from build123d import *

# Parameters (mm, degrees)
BOSS_EXTRUDE1_START  = 46
SKETCH1_W            = 40
SKETCH1_H            = 10
BOSS_EXTRUDE1_DEPTH  = 28
BOSS_EXTRUDE2_START  = 48.4
SKETCH2_W            = 35.2
SKETCH2_H            = 12
BOSS_EXTRUDE2_DEPTH  = 23.2
BOSS_EXTRUDE3_START  = 50
SKETCH3_R            = 3
BOSS_EXTRUDE3_DEPTH  = 10
BOSS_EXTRUDE4_START  = 50
SKETCH4_R            = 3
BOSS_EXTRUDE4_DEPTH  = 10
BOSS_EXTRUDE5_START  = 50
SKETCH5_R            = 3
BOSS_EXTRUDE5_DEPTH  = 10
BOSS_EXTRUDE6_START  = 50
SKETCH6_R            = 3
BOSS_EXTRUDE6_DEPTH  = 10
BOSS_EXTRUDE7_START  = 50
SKETCH7_R            = 3
BOSS_EXTRUDE7_DEPTH  = 10
BOSS_EXTRUDE8_START  = 50
SKETCH8_R            = 3
BOSS_EXTRUDE8_DEPTH  = 10
BOSS_EXTRUDE9_START  = 50
SKETCH9_R            = 3
BOSS_EXTRUDE9_DEPTH  = 10
BOSS_EXTRUDE10_START = 50
SKETCH10_R           = 3
BOSS_EXTRUDE10_DEPTH = 10
BOSS_EXTRUDE11_START = 49
SKETCH11_R           = 1
BOSS_EXTRUDE11_DEPTH = 9.5
BOSS_EXTRUDE12_START = 49
SKETCH12_R           = 1
BOSS_EXTRUDE12_DEPTH = 9.5
BOSS_EXTRUDE13_START = 49
SKETCH13_R           = 1
BOSS_EXTRUDE13_DEPTH = 9.5
BOSS_EXTRUDE14_START = 49
SKETCH14_R           = 1
BOSS_EXTRUDE14_DEPTH = 9.5
BOSS_EXTRUDE15_START = 51.5
SKETCH15_R           = 1
BOSS_EXTRUDE15_DEPTH = 9.5
BOSS_EXTRUDE16_START = 51.5
SKETCH16_R           = 1
BOSS_EXTRUDE16_DEPTH = 9.5
BOSS_EXTRUDE17_START = 51.5
SKETCH17_R           = 1
BOSS_EXTRUDE17_DEPTH = 9.5
BOSS_EXTRUDE18_START = 51.5
SKETCH18_R           = 1
BOSS_EXTRUDE18_DEPTH = 9.5


with BuildPart() as part:
    # Sketch1 → Boss-Extrude1 (new body)
    with BuildSketch(Plane.XY.offset(BOSS_EXTRUDE1_START)):
        with Locations((0, 55)):
            Rectangle(SKETCH1_W, SKETCH1_H)
    extrude(amount=BOSS_EXTRUDE1_DEPTH)


with BuildPart() as body_2:
    # Sketch2 → Boss-Extrude2 (new body)
    with BuildSketch(Plane.XY.offset(BOSS_EXTRUDE2_START)):
        with Locations((0, 55)):
            Rectangle(SKETCH2_W, SKETCH2_H)
    extrude(amount=BOSS_EXTRUDE2_DEPTH)


with BuildPart() as part_1:
    add(part.part)

    # Combine1: cut body 2
    add(body_2.part, mode=Mode.SUBTRACT)

    # Sketch3 → Boss-Extrude3 (add)
    with BuildSketch(Plane(origin=(0, 0, 0), x_dir=(1, 0, 0), z_dir=(0, 1, 0)).offset(BOSS_EXTRUDE3_START)):
        with Locations((-15, -50.5)):
            Circle(SKETCH3_R)
    extrude(amount=BOSS_EXTRUDE3_DEPTH)

    # Sketch4 → Boss-Extrude4 (add)
    with BuildSketch(Plane(origin=(0, 0, 0), x_dir=(1, 0, 0), z_dir=(0, 1, 0)).offset(BOSS_EXTRUDE4_START)):
        with Locations((-15, -69.5)):
            Circle(SKETCH4_R)
    extrude(amount=BOSS_EXTRUDE4_DEPTH)

    # Sketch5 → Boss-Extrude5 (add)
    with BuildSketch(Plane(origin=(0, 0, 0), x_dir=(1, 0, 0), z_dir=(0, 1, 0)).offset(BOSS_EXTRUDE5_START)):
        with Locations((15, -50.5)):
            Circle(SKETCH5_R)
    extrude(amount=BOSS_EXTRUDE5_DEPTH)

    # Sketch6 → Boss-Extrude6 (add)
    with BuildSketch(Plane(origin=(0, 0, 0), x_dir=(1, 0, 0), z_dir=(0, 1, 0)).offset(BOSS_EXTRUDE6_START)):
        with Locations((15, -69.5)):
            Circle(SKETCH6_R)
    extrude(amount=BOSS_EXTRUDE6_DEPTH)

    # Sketch7 → Boss-Extrude7 (add)
    with BuildSketch(Plane(origin=(0, 0, 0), x_dir=(1, 0, 0), z_dir=(0, 1, 0)).offset(BOSS_EXTRUDE7_START)):
        with Locations((-6, -50)):
            Circle(SKETCH7_R)
    extrude(amount=BOSS_EXTRUDE7_DEPTH)

    # Sketch8 → Boss-Extrude8 (add)
    with BuildSketch(Plane(origin=(0, 0, 0), x_dir=(1, 0, 0), z_dir=(0, 1, 0)).offset(BOSS_EXTRUDE8_START)):
        with Locations((-6, -70)):
            Circle(SKETCH8_R)
    extrude(amount=BOSS_EXTRUDE8_DEPTH)

    # Sketch9 → Boss-Extrude9 (add)
    with BuildSketch(Plane(origin=(0, 0, 0), x_dir=(1, 0, 0), z_dir=(0, 1, 0)).offset(BOSS_EXTRUDE9_START)):
        with Locations((6, -50)):
            Circle(SKETCH9_R)
    extrude(amount=BOSS_EXTRUDE9_DEPTH)

    # Sketch10 → Boss-Extrude10 (add)
    with BuildSketch(Plane(origin=(0, 0, 0), x_dir=(1, 0, 0), z_dir=(0, 1, 0)).offset(BOSS_EXTRUDE10_START)):
        with Locations((6, -70)):
            Circle(SKETCH10_R)
    extrude(amount=BOSS_EXTRUDE10_DEPTH)


with BuildPart() as body_2_2:
    # Sketch11 → Boss-Extrude11 (new body)
    with BuildSketch(Plane(origin=(0, 0, 0), x_dir=(1, 0, 0), z_dir=(0, 1, 0)).offset(BOSS_EXTRUDE11_START)):
        with Locations(Location((-15, -50.5, 0), (0, 0, 270))):
            Circle(SKETCH11_R)
    extrude(amount=BOSS_EXTRUDE11_DEPTH)


with BuildPart() as part_2:
    add(part_1.part)

    # Combine2: cut body 2 2
    add(body_2_2.part, mode=Mode.SUBTRACT)


with BuildPart() as body_2_3:
    # Sketch12 → Boss-Extrude12 (new body)
    with BuildSketch(Plane(origin=(0, 0, 0), x_dir=(1, 0, 0), z_dir=(0, 1, 0)).offset(BOSS_EXTRUDE12_START)):
        with Locations(Location((-15, -69.5, 0), (0, 0, 270))):
            Circle(SKETCH12_R)
    extrude(amount=BOSS_EXTRUDE12_DEPTH)


with BuildPart() as part_3:
    add(part_2.part)

    # Combine3: cut body 2 3
    add(body_2_3.part, mode=Mode.SUBTRACT)


with BuildPart() as body_2_4:
    # Sketch13 → Boss-Extrude13 (new body)
    with BuildSketch(Plane(origin=(0, 0, 0), x_dir=(1, 0, 0), z_dir=(0, 1, 0)).offset(BOSS_EXTRUDE13_START)):
        with Locations(Location((15, -50.5, 0), (0, 0, 270))):
            Circle(SKETCH13_R)
    extrude(amount=BOSS_EXTRUDE13_DEPTH)


with BuildPart() as part_4:
    add(part_3.part)

    # Combine4: cut body 2 4
    add(body_2_4.part, mode=Mode.SUBTRACT)


with BuildPart() as body_2_5:
    # Sketch14 → Boss-Extrude14 (new body)
    with BuildSketch(Plane(origin=(0, 0, 0), x_dir=(1, 0, 0), z_dir=(0, 1, 0)).offset(BOSS_EXTRUDE14_START)):
        with Locations(Location((15, -69.5, 0), (0, 0, 270))):
            Circle(SKETCH14_R)
    extrude(amount=BOSS_EXTRUDE14_DEPTH)


with BuildPart() as part_5:
    add(part_4.part)

    # Combine5: cut body 2 5
    add(body_2_5.part, mode=Mode.SUBTRACT)


with BuildPart() as body_2_6:
    # Sketch15 → Boss-Extrude15 (new body)
    with BuildSketch(Plane(origin=(0, 0, 0), x_dir=(1, 0, 0), z_dir=(0, 1, 0)).offset(BOSS_EXTRUDE15_START)):
        with Locations(Location((-6, -50, 0), (0, 0, 270))):
            Circle(SKETCH15_R)
    extrude(amount=BOSS_EXTRUDE15_DEPTH)


with BuildPart() as part_6:
    add(part_5.part)

    # Combine6: cut body 2 6
    add(body_2_6.part, mode=Mode.SUBTRACT)


with BuildPart() as body_2_7:
    # Sketch16 → Boss-Extrude16 (new body)
    with BuildSketch(Plane(origin=(0, 0, 0), x_dir=(1, 0, 0), z_dir=(0, 1, 0)).offset(BOSS_EXTRUDE16_START)):
        with Locations(Location((-6, -70, 0), (0, 0, 270))):
            Circle(SKETCH16_R)
    extrude(amount=BOSS_EXTRUDE16_DEPTH)


with BuildPart() as part_7:
    add(part_6.part)

    # Combine7: cut body 2 7
    add(body_2_7.part, mode=Mode.SUBTRACT)


with BuildPart() as body_2_8:
    # Sketch17 → Boss-Extrude17 (new body)
    with BuildSketch(Plane(origin=(0, 0, 0), x_dir=(1, 0, 0), z_dir=(0, 1, 0)).offset(BOSS_EXTRUDE17_START)):
        with Locations(Location((6, -50, 0), (0, 0, 270))):
            Circle(SKETCH17_R)
    extrude(amount=BOSS_EXTRUDE17_DEPTH)


with BuildPart() as part_8:
    add(part_7.part)

    # Combine8: cut body 2 8
    add(body_2_8.part, mode=Mode.SUBTRACT)


with BuildPart() as body_2_9:
    # Sketch18 → Boss-Extrude18 (new body)
    with BuildSketch(Plane(origin=(0, 0, 0), x_dir=(1, 0, 0), z_dir=(0, 1, 0)).offset(BOSS_EXTRUDE18_START)):
        with Locations(Location((6, -70, 0), (0, 0, 270))):
            Circle(SKETCH18_R)
    extrude(amount=BOSS_EXTRUDE18_DEPTH)


with BuildPart() as part_9:
    add(part_8.part)

    # Combine9: cut body 2 9
    add(body_2_9.part, mode=Mode.SUBTRACT)


solid = part_9.part
Input: part model. Units: mm. Frame: model coordinates. A direction names the side the tool comes from. Coordinates: 2 decimals unless noted, no trailing zeros. Loops run counter-clockwise (first coordinate to the right, second up) from the corner with the lowest first, then second, coordinate; pieces in that order, holes last. Notation, with made-up numbers: (18, -16.75) -> (45, -16.75) arc R13 cw to (45, 4.25) -> close; hole circle Ø7 at (89, -22.5). An arc over 180 degrees is marked (long way). Write item = value, one per line. Start each with the question number.
Item 1: Cut plane C-C, the plane x = -11.5. Return loops of the section in (y, z), plus the area to 3 significant figures.
Item 2: Mould query, pull axis X, two halves, no side actions, for faces 5 (the face through (-5, 50, 50)), 6 (the face through (-11, 55, 48.4)), 7 (the face through (-20, 55, 60)). Classes: pulls with the +X half, pulls with the -X half, needs draft (parallel to the pull), parting line crosses it, or undercut.
Item 3: Cut plane A-A, the plane x = 6. Return loops of the section in (y, z).
Item 4: Reachability of faces 1 (the face through (-15, 58.5, 50)), 2 (the face through (6, 56, 69)), 3 (the face through (-4.7, 60, 50.5)), 4 (the face through (0, 55, 71.6)) from +Z, -Z, +X, -X, +Y, -Y: full face, straight path, thin tool, end or side. Return the list, or none.
Item 5: Material intervals for line 1 (Z direction, x = 15, y = 55.25); line 2 (Z direction, x = 6, y = 54.25); line 3 (Z direction, x = -11, y = 53.25), sorted ascending.
Item 6: First-contact query: P1, Ø2, axis at x = 14.5, z = 69, coming from the -Y side; P2, Ø8, axis at x = 9.5, z = 57.5, coming from the -Y side; P3, Ø1.6, axis at x = -6, z = 50, coming from the +Y side. Flat tips, straight axial feed; report the tip coordinate or a pass-through.
Item 7: Cut plane B-B, the plane z = 61.75. Return loops of the section in (x, y), plus the area to 3 significant figures.
Item 8: Cut plane D-D, the plane y = 53. Count the separate pieces of the cut face and the enclosed holes in it, plus the area to 3 significant figures.
Ans:
q1.outline = (50, 46) -> (60, 46) -> (60, 48.4) -> (50, 48.4) -> close; (50, 71.6) -> (60, 71.6) -> (60, 74) -> (50, 74) -> close
q1.area = 48.0 mm²
q2.face_5 = needs draft
q2.face_6 = undercut
q2.face_7 = pulls with the -X half
q3.outline = (50, 46) -> (60, 46) -> (60, 49) -> (51.5, 49) -> (51.5, 51) -> (60, 51) -> (60, 53) -> (50, 53) -> close; (50, 67) -> (60, 67) -> (60, 69) -> (51.5, 69) -> (51.5, 71) -> (60, 71) -> (60, 74) -> (50, 74) -> close
q4.face_1 = -Y
q4.face_2 = +Y
q4.face_3 = +Z, -Z, +X, -X, +Y
q4.face_4 = +Y, -Y
q5.line_1 = 46 to 49.5, 51.5 to 53.5, 66.5 to 68.5, 70.5 to 74
q5.line_2 = 46 to 49, 51 to 53, 67 to 69, 71 to 74
q5.line_3 = 46 to 48.4, 71.6 to 74
q6.P1 = 50
q6.P2 = through
q6.P3 = 51.5
q7.outline = (-20, 50) -> (-17.6, 50) -> (-17.6, 60) -> (-20, 60) -> close; (17.6, 50) -> (20, 50) -> (20, 60) -> (17.6, 60) -> close
q7.area = 48.0 mm²
q8.separate_pieces = 1
q8.enclosed_holes = 13
q8.area = 470 mm²
